Read the model definition and answer for the solid it produces. Units are mm, in the model's axes. A direction names the side the tool comes from. Coordinates: 2 decimals unless noted, no trailing zeros. Write each loop counter-clockwise with the first axis right and the second up, starting at its lowest first coordinate (ties: lowest second). Pieces come first, ordered by that corner, then holes.
Item 1: Straight lines are drawn through the part: probe 1 along Z at (x, y) = (7.5, 41.5); probe 2 along Y at (x, z) = (-47, 3.5); probe 3 along X at (y, z) = (43.5, 31.5). For each, find the intervals that lie inside material, in ascending order.
Item 2: A tool of negligible diameter and unlimited length cuts with its end or side. For faces 4 (the face through (-51.52, -3.27, 32.98)), 5 (the face through (49.493, -3.364, 32.984)), 6 (the face through (34.669, 7, 3)), 7 (the face through (49.561, 43.482, 32.984)), from which of +Z, -Z, +X, -X, +Y, -Y can it reach the whole face along a straight path? Write none if from no direction.
Item 3: Section D-D (z = 26) is taken. Give the vertices of the cut face in (x, y).
Item 4: Section C-C (x = 38.5) is taken. Give the vertices of the cut face in (y, z), then the cut area to 3 significant figures.
Item 5: Section B-B (z = 4) is taken. Give the vertices of the cut face in (x, y), then the cut area to 3 significant figures.
Item 6: Section A-A (y = 39) is taken. Give the vertices of the cut face in (x, z), then the cut area to 3 significant figures.
Item 7: Determine the mould class of faces 1 (the face through (-2, 20, 0)), 2 (the face through (29.79, 10.69, 2.5)), 3 (the face through (-2, 20, 30.48)) for opening direction Z: released by +Z, released by -Z, zero draft, split by the parting line, or undercut.
Item 8: Each of these flat-tipped pins is pushed along its axis until it touches: P1, Ø2.5, axis at y = 21, z = 32, coming from the +X side; P2, Ø12, axis at y = 29, z = 15.5, coming from the +X side; P3, Ø2.5, axis at x = -13, z = 3.5, coming from the -Y side; P4, Ø3, axis at y = 7.5, z = 1.5, coming from the -X side. Where does it stop, or does it pass through?
from build123d import *

# Parameters (mm, degrees)
F1_DEPTH = 5.08
F3_DEPTH = 25.4
F5_DEPTH = 5.08
F7_DEPTH = 5.08


with BuildPart() as f1:
    # F0 (on Top) → F1 (new body)
    with BuildSketch(Plane.XY):
        Polygon((47.303539, 46.30276), (-48.649952, 46.30276), (-54.208234, 40.744482), (-54.208234, 0), (-49.235035, -6.582176), (47.303539, -6.582176), (51.984198, 0), (51.984198, 40.744482), align=None)
    extrude(amount=F1_DEPTH)

    # F2 (on face) → F3 (join)
    with BuildSketch(Plane.XY.offset(5.08)):
        Polygon((-48.649952, 46.30276), (-49.959227, 44.993486), (-48.649952, 43.68421), (-47.324431, 45.00973), (-47.324431, 46.30276), align=None)
    extrude(amount=F3_DEPTH)

    # F4 (on face) → F5 (join)
    with BuildSketch(Plane.XY.offset(30.48)):
        Polygon((47.10824, 46.30276), (-48.649952, 46.30276), (-54.313436, 40.739778), (-54.313436, 0), (-48.649952, -6.634823), (47.10824, -6.634823), (51.945787, 0), (51.945787, 40.739778), align=None)
    extrude(amount=F5_DEPTH)

    # F6 (on face) → F7 (cut)
    with BuildSketch(Plane(origin=(0, 0, 0), x_dir=(1, 0, 0), z_dir=(0, 0, -1))):
        Polygon((34.669146, -9.18433), (34.669146, -5.294323), (31.111144, -2.706686), (28.497104, -5.180843), (28.497104, -9.18433), (31.111144, -12.234045), align=None)
    extrude(amount=-F7_DEPTH, mode=Mode.SUBTRACT)


solid = f1.part
Established:
1. probe 1: z = 0 to 5.08, 30.48 to 35.56
1. probe 2: y = -6.58 to 46.3
1. probe 3: x = -51.5 to 49.55
2. face 4: +Z, -X, -Y
2. face 5: +Z, +X, -Y
2. face 6: -Z
2. face 7: +Z, +X, +Y
3. outline: (-49.96, 44.99) - (-48.65, 43.68) - (-47.32, 45.01) - (-47.32, 46.3) - (-48.65, 46.3) - close
4. outline: (-6.63, 30.48) - (46.3, 30.48) - (46.3, 35.56) - (-6.63, 35.56) - close; (-6.58, 0) - (46.3, 0) - (46.3, 5.08) - (-6.58, 5.08) - close
4. area: 538 mm2
5. outline: (-54.21, 0) - (-49.24, -6.58) - (47.3, -6.58) - (51.98, 0) - (51.98, 40.74) - (47.3, 46.3) - (-48.65, 46.3) - (-54.21, 40.74) - close; hole (28.5, 5.18) - (31.11, 2.71) - (34.67, 5.29) - (34.67, 9.18) - (31.11, 12.23) - (28.5, 9.18) - close
5. area: 5,510 mm2
6. outline: (-54.31, 30.48) - (51.95, 30.48) - (51.95, 35.56) - (-54.31, 35.56) - close; (-54.21, 0) - (51.98, 0) - (51.98, 5.08) - (-54.21, 5.08) - close
6. area: 1,080 mm2
7. face 1: released by -Z
7. face 2: zero draft
7. face 3: undercut
8. P1: stops at x = 51.95
8. P2: passes through
8. P3: stops at y = -6.58
8. P4: stops at x = -54.21
